Build history of the part. All positions in model axes, mm. Give positions to 0.01 mm unless a question says otherwise; leave off trailing zeros. Loops run counter-clockwise (first coordinate to the right, second up) from the corner with the lowest first, then second, coordinate; pieces in that order, holes last.
1) Two-plate mould, pull along Y, no slides. Class faces 1 (the cylindrical face through (1.57, -237.95, -63.06)), 2 (the cylindrical face through (1.57, -237.95, 63.94)), 3 (the cylindrical face through (1.565, 25.395, 0.485)), 4 (the flat face through (3.175, -143, -1)): +Y half, -Y half, draft (parallel to the pull), parting line (faces both ways), or undercut.
2) Band-saw the part on C-C on y = -241.3. List the corners of the cut face in (x, z) (3 decimals).
3) Wall check: line 1 (Z direction, x = 2.15, y = -241.3); line 2 (Z direction, x = 0.55, y = 4); line 3 (Y direction, x = 2.6, z = -6.5). Give the ranges that are in metal, low to high.
4) Band-saw the part on A-A on z = 0. List the corners of the cut face in (x, y) (1 decimal), then the cut area to 3 significant figures.
5) Band-saw the part on D-D on y = 0. List the corners of the cut face in (x, z) (1 decimal), then the cut area to 3 significant figures.
6) Band-saw the part on B-B on x = 0.7. List the corners of the cut face in (y, z) (1 decimal).
```python
from build123d import *

# Parameters (mm, degrees)
SKETCH1_R           = 14.2875
SKETCH1_R_2         = 3.3782
BOSS_EXTRUDE1_DEPTH = 3.175


with BuildPart() as part:
    # Sketch1 → Boss-Extrude1 (new body)
    with BuildSketch(Plane(origin=(0, 0, 0), x_dir=(0, 0, -1), z_dir=(1, 0, 0))):
        with BuildLine():
            Line((-75.93043495, -238.69725396), (-24.860869901, 5.205492079))
            ThreePointArc((-24.860869901, 5.205492079), (0, 25.4), (24.860869901, 5.205492079))
            Line((24.860869901, 5.205492079), (75.93043495, -238.69725396))
            ThreePointArc((75.93043495, -238.69725396), (73.357608095, -249.307344294), (63.5, -254))
            Line((63.5, -254), (-63.5, -254))
            ThreePointArc((-63.5, -254), (-73.357608095, -249.307344294), (-75.93043495, -238.69725396))
        make_face()
        Circle(SKETCH1_R, mode=Mode.SUBTRACT)
        with Locations((-63.5, -241.3)):
            Circle(SKETCH1_R_2, mode=Mode.SUBTRACT)
        with Locations((0, -241.3)):
            Circle(SKETCH1_R_2, mode=Mode.SUBTRACT)
        with Locations((63.5, -241.3)):
            Circle(SKETCH1_R_2, mode=Mode.SUBTRACT)
    extrude(amount=BOSS_EXTRUDE1_DEPTH)


solid = part.part
```
Findings below:
1. face 1: undercut
1. face 2: undercut
1. face 3: +Y half
1. face 4: draft
2. outline: (0, -76.2) - (3.175, -76.2) - (3.175, -66.878) - (0, -66.878) - close; (0, -60.122) - (3.175, -60.122) - (3.175, -3.378) - (0, -3.378) - close; (0, 3.378) - (3.175, 3.378) - (3.175, 60.122) - (0, 60.122) - close; (0, 66.878) - (3.175, 66.878) - (3.175, 76.2) - (0, 76.2) - close
3. line 1: z = -76.2 to -66.88, -60.12 to -3.38, 3.38 to 60.12, 66.88 to 76.2
3. line 2: z = -25.11 to -13.72, 13.72 to 25.11
3. line 3: y = -254 to -12.72, 12.72 to 24.55
4. outline: (0, -254) - (3.2, -254) - (3.2, -244.7) - (0, -244.7) - close; (0, -237.9) - (3.2, -237.9) - (3.2, -14.3) - (0, -14.3) - close; (0, 14.3) - (3.2, 14.3) - (3.2, 25.4) - (0, 25.4) - close
4. area: 775 mm2
5. outline: (0, -26) - (3.2, -26) - (3.2, -14.3) - (0, -14.3) - close; (0, 14.3) - (3.2, 14.3) - (3.2, 26) - (0, 26) - close
5. area: 74.1 mm2
6. outline: (-254, -63.5) arc R12.7 ccw to (-238.7, -75.9) - (5.2, -24.9) arc R25.4 ccw to (5.2, 24.9) - (-238.7, 75.9) arc R12.7 ccw to (-254, 63.5) - close; hole circle Ø6.8 at (-241.3, -63.5); hole circle Ø6.8 at (-241.3, 0); hole circle Ø6.8 at (-241.3, 63.5); hole circle Ø28.6 at (0, 0)
